Geometry check sheet. Reference: the model listing, model coordinates, mm. A direction names the side the tool comes from. Round coordinates to 2 decimals unless told otherwise and drop trailing zeros. Write each loop counter-clockwise with the first axis right and the second up, starting at its lowest first coordinate (ties: lowest second). Pieces come first, ordered by that corner, then holes. Notation, with made-up numbers: (81, 71.25) - (118, 71.25) arc R25 cw to (118, 83.25) - close; hole circle Ø4 at (15.25, 68). An arc over 180 degrees is marked (long way). Return JSON: item names as keys, results as strings.
```python
from build123d import *

# Parameters (mm, degrees)
F2_DEPTH = 24
F3_DEPTH = 21
F4_DEPTH = 15.5
F5_DEPTH = 12
F6_DEPTH = 4
F7_R     = 1.3
F8_DEPTH = 11.001


with BuildPart() as f2:
    # F1 (on Top) → F2 (new body)
    with BuildSketch(Plane.XY):
        with BuildLine():
            Line((11, 11), (0, 11))
            Line((0, 11), (0, 8))
            ThreePointArc((0, 8), (5.6568542495, 5.6568542495), (8, 0))
            ThreePointArc((8, 0), (5.6568542495, -5.6568542495), (0, -8))
            Line((0, -8), (0, -11))
            Line((0, -11), (11, -11))
            Line((11, -11), (11, 11))
        make_face()
    extrude(amount=F2_DEPTH)

    # F1 (on Top) → F3 (join)
    with BuildSketch(Plane.XY):
        with BuildLine():
            ThreePointArc((8, 0), (5.6568542495, 5.6568542495), (0, 8))
            Line((0, 8), (0, 6))
            ThreePointArc((0, 6), (4.2426406871, 4.2426406871), (6, 0))
            ThreePointArc((6, 0), (4.2426406871, -4.2426406871), (0, -6))
            Line((0, -6), (0, -8))
            ThreePointArc((0, -8), (5.6568542495, -5.6568542495), (8, 0))
        make_face()
    extrude(amount=F3_DEPTH)

    # F1 (on Top) → F4 (cut)
    with BuildSketch(Plane.XY):
        with BuildLine():
            ThreePointArc((8, 0), (5.6568542495, 5.6568542495), (0, 8))
            Line((0, 8), (0, 6))
            ThreePointArc((0, 6), (4.2426406871, 4.2426406871), (6, 0))
            ThreePointArc((6, 0), (4.2426406871, -4.2426406871), (0, -6))
            Line((0, -6), (0, -8))
            ThreePointArc((0, -8), (5.6568542495, -5.6568542495), (8, 0))
        make_face()
        with BuildLine():
            Line((0, 6), (0, 8))
            ThreePointArc((0, 8), (-8, 0), (0, -8))
            Line((0, -8), (0, -6))
            ThreePointArc((0, -6), (-6, 0), (0, 6))
        make_face()
    extrude(amount=F4_DEPTH, mode=Mode.SUBTRACT)

    # F1 (on Top) → F5 (join)
    with BuildSketch(Plane.XY):
        with BuildLine():
            ThreePointArc((8, 0), (5.6568542495, 5.6568542495), (0, 8))
            Line((0, 8), (0, 6))
            ThreePointArc((0, 6), (4.2426406871, 4.2426406871), (6, 0))
            ThreePointArc((6, 0), (4.2426406871, -4.2426406871), (0, -6))
            Line((0, -6), (0, -8))
            ThreePointArc((0, -8), (5.6568542495, -5.6568542495), (8, 0))
        make_face()
        with BuildLine():
            ThreePointArc((6, 0), (4.2426406871, 4.2426406871), (0, 6))
            Line((0, 6), (0, 2.25))
            ThreePointArc((0, 2.25), (1.5909902577, 1.5909902577), (2.25, 0))
            ThreePointArc((2.25, 0), (1.5909902577, -1.5909902577), (0, -2.25))
            Line((0, -2.25), (0, -6))
            ThreePointArc((0, -6), (4.2426406871, -4.2426406871), (6, 0))
        make_face()
        with BuildLine():
            ThreePointArc((2.25, 0), (1.5909902577, 1.5909902577), (0, 2.25))
            Line((0, 2.25), (0, 1))
            ThreePointArc((0, 1), (0.7071067812, 0.7071067812), (1, 0))
            ThreePointArc((1, 0), (0.7071067812, -0.7071067812), (0, -1))
            Line((0, -1), (0, -2.25))
            ThreePointArc((0, -2.25), (1.5909902577, -1.5909902577), (2.25, 0))
        make_face()
    extrude(amount=F5_DEPTH)

    # F1 (on Top) → F6 (cut)
    with BuildSketch(Plane.XY):
        with BuildLine():
            ThreePointArc((2.25, 0), (1.5909902577, 1.5909902577), (0, 2.25))
            Line((0, 2.25), (0, 1))
            ThreePointArc((0, 1), (0.7071067812, 0.7071067812), (1, 0))
            ThreePointArc((1, 0), (0.7071067812, -0.7071067812), (0, -1))
            Line((0, -1), (0, -2.25))
            ThreePointArc((0, -2.25), (1.5909902577, -1.5909902577), (2.25, 0))
        make_face()
        with BuildLine():
            Line((0, 1), (0, 2.25))
            ThreePointArc((0, 2.25), (-2.25, 0), (0, -2.25))
            Line((0, -2.25), (0, -1))
            ThreePointArc((0, -1), (-1, 0), (0, 1))
        make_face()
    extrude(amount=F6_DEPTH, mode=Mode.SUBTRACT)

    # F7 (on face) → F8 (cut, through all)
    with BuildSketch(Plane(origin=(0, 0, 0), x_dir=(0, -1, 0), z_dir=(-1, 0, 0))):
        with Locations((-7.5, 18.25)):
            Circle(F7_R)
        with Locations((7.5, 18.25)):
            Circle(F7_R)
        with Locations((7.5, 3.25)):
            Circle(F7_R)
        with Locations((-7.5, 3.25)):
            Circle(F7_R)
    extrude(amount=-F8_DEPTH, mode=Mode.SUBTRACT)


solid = f2.part
```
(1) Release check for a two-part mould opening along Z. For faces 5 (the face through (9, 0, 24)), 6 (the face through (11, 0, 12)), 7 (the face through (5.42, -8.7, 17.75)) record: pulls with the +Z half, pulls with the -Z half, needs draft (parallel to the pull), parting line crosses it, or undercut.
Response values:
{"face 5": "pulls with the +Z half", "face 6": "needs draft", "face 7": "undercut"}
(2) Section check D-D, the plane z = 3.25. Enter the section's corners in (x, y).
Response values:
{"outline": "(0, -11) - (11, -11) - (11, -8.8) - (0, -8.8) - close; (0, -6.2) - (11, -6.2) - (11, 6.2) - (0, 6.2) - (0, 2.25) arc R2.25 cw to (0, -2.25) - close; (0, 8.8) - (11, 8.8) - (11, 11) - (0, 11) - close"}
(3) Material ranges on line 1 along Z through (x, y) = (5.75, -7.5); line 2 along Z through (x, y) = (7.5, -2); line 3 along Y through (x, z) = (2.25, 18), recorded low to high. Write a range as [from, to].
Response values:
{"line 1": "z = [0, 1.95], [4.55, 16.95], [19.55, 24]", "line 2": "z = [0, 12], [15.5, 21]", "line 3": "y = [-11, -8.78], [-6.22, -5.56], [5.56, 6.22], [8.78, 11]"}
(4) Section check A-A, the plane z = 18.25. Enter the section's corners in (x, y).
Response values:
{"outline": "(0, -11) - (11, -11) - (11, -8.8) - (0, -8.8) - close; (0, -6.2) - (11, -6.2) - (11, 6.2) - (0, 6.2) - (0, 6) arc R6 cw to (0, -6) - close; (0, 8.8) - (11, 8.8) - (11, 11) - (0, 11) - close"}
(5) Section check B-B, the plane x = 0.5. Enter the section's corners in (y, z).
Response values:
{"outline": "(-11, 0) - (-2.19, 0) - (-2.19, 4) - (-0.87, 4) - (-0.87, 12) - (-7.98, 12) - (-7.98, 15.5) - (-5.98, 15.5) - (-5.98, 21) - (-7.98, 21) - (-7.98, 24) - (-11, 24) - close; (0.87, 4) - (2.19, 4) - (2.19, 0) - (11, 0) - (11, 24) - (7.98, 24) - (7.98, 21) - (5.98, 21) - (5.98, 15.5) - (7.98, 15.5) - (7.98, 12) - (0.87, 12) - close; hole circle Ø2.6 at (-7.5, 3.25); hole circle Ø2.6 at (-7.5, 18.25); hole circle Ø2.6 at (7.5, 3.25); hole circle Ø2.6 at (7.5, 18.25)"}
(6) Section check C-C, the plane y = 7.5. Enter the section's corners in (x, z).
Response values:
{"outline": "(0, 0) - (11, 0) - (11, 1.95) - (0, 1.95) - close; (0, 4.55) - (11, 4.55) - (11, 16.95) - (0, 16.95) - (0, 15.5) - (2.78, 15.5) - (2.78, 12) - (0, 12) - close; (0, 19.55) - (11, 19.55) - (11, 24) - (2.78, 24) - (2.78, 21) - (0, 21) - close"}
(7) Access from +Z, -Z, +X, -X, +Y, -Y to the whole of each face (thin tool, end or side, straight path). Record for faces 1 (the face through (5.423, 6.9, 17.097)), 2 (the face through (6.4, -0.6, 21)), 3 (the face through (6.4, -0.6, 15.5)), 4 (the face through (1.4, 0, 4)).
Response values:
{"face 1": "+X, -X", "face 2": "+Z, -X", "face 3": "-X", "face 4": "-Z, -X"}
(8) Gauge pin test, flat ends, axial feed: pin 1 (2 mm diameter, centred on y = -7.5, z = 18.25, fed in from -X); pin 2 (4 mm diameter, centred on x = 4, y = 3.5, fed in from +Z); pin 3 (2.5 mm diameter, centred on x = 3, y = -3, fed in from +Z). Record the tip position at first contact, or that the pin passes through.
Response values:
{"pin 1": "passes through", "pin 2": "stops at z = 21", "pin 3": "stops at z = 12"}
